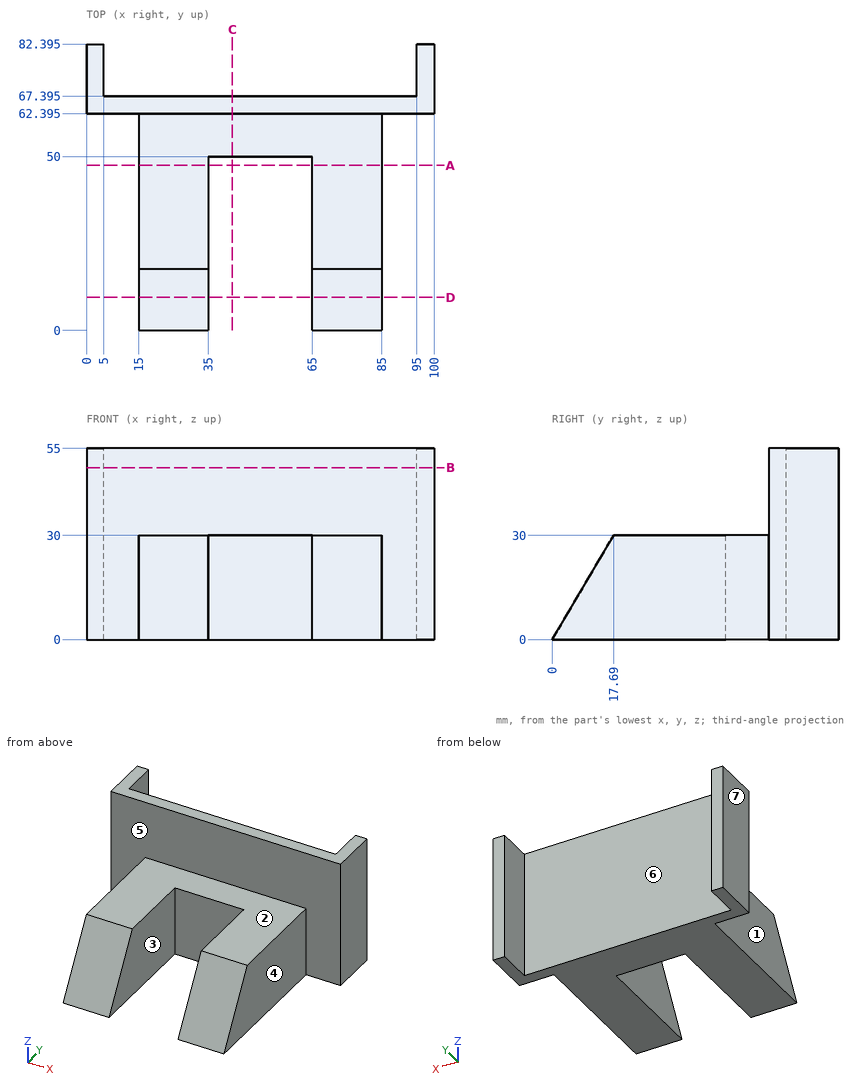
Here's the drawing with two shaded views (mm, measured from the low corner). I have some questions. A direction names the side the tool comes from. Round coordinates to 2 decimals unless told otherwise and drop trailing zeros. Loops run counter-clockwise (first coordinate to the right, second up) from the corner with the lowest first, then second, coordinate; pieces in that order, holes last. Notation, with made-up numbers: (79, 76) -> (129, 76) arc R19 ccw to (129, 86) -> close; hole circle Ø2 at (0, 48). An arc over 180 degrees is marked (long way). Answer as CSV lines item,"result". Start each with the question number.
1. Imagine slicing it at B-B on z = 49.5. Write out the boundary of the cut face in (x, y) (3 decimals).
2. I need wall thicknesses on probe 1 along X at (y, z) = (72, 46.5); probe 2 along X at (y, z) = (17, 23); probe 3 along Y at (x, z) = (61.5, 15) (3 decimals). Which ranges of each line are inside material? Lowest first, please. Write a range as from..to.
3. Imagine slicing it at C-C on x = 42. Write out the boundary of the cut face in (y, z) (3 decimals).
4. Imagine slicing it at A-A on y = 47.5. Write out the boundary of the cut face in (x, z).
5. If we mould it in two halves opening along X, with no side actions, what happens to the marked faces 5, 6 and 7? For each: pulls with the +X half, pulls with the -X half, needs draft (parallel to the pull), parting line crosses it, or undercut.
6. Imagine slicing it at D-D on y = 9.5. Write out the boundary of the cut face in (x, z), plus the area to 3 significant figures.
7. I'm going to push flat-ended pins straight in: P1, Ø16.5, axis at x = 54, z = 35.5, coming from the +Y side (3 decimals); P2, Ø8, axis at x = 71, z = 19, coming from the -Y side (3 decimals); P3, Ø24, axis at y = 15, z = 12.5, coming from the -X side. Where does each tip first touch, or does it pass through?
8. For the marked faces 1, 2, 3 and 4, which set-ups out of +Z, -Z, +X, -X, +Y, -Y let a thin tool reach every point of the face, with its end or its side?
Solution:
1,outline,"(0, 62.395) -> (100, 62.395) -> (100, 82.395) -> (95, 82.395) -> (95, 67.395) -> (5, 67.395) -> (5, 82.395) -> (0, 82.395) -> close"
2,probe 1,"0..5, 95..100"
2,probe 2,"15..35, 65..85"
2,probe 3,"50..67.395"
3,outline,"(50, 0) -> (67.395, 0) -> (67.395, 55) -> (62.395, 55) -> (62.395, 30) -> (50, 30) -> close"
4,outline,"(15, 0) -> (35, 0) -> (35, 30) -> (15, 30) -> close; (65, 0) -> (85, 0) -> (85, 30) -> (65, 30) -> close"
5,face 5,"needs draft"
5,face 6,"undercut"
5,face 7,"pulls with the -X half"
6,outline,"(15, 0) -> (35, 0) -> (35, 16.11) -> (15, 16.11) -> close; (65, 0) -> (85, 0) -> (85, 16.11) -> (65, 16.11) -> close"
6,area,"644 mm²"
7,P1,"y = 67.395"
7,P2,"y = 8.845"
7,P3,"x = 15"
8,face 1,"+Z, -Z, -X, -Y"
8,face 2,"+Z, +X, -X, -Y"
8,face 3,"+Z, -Z, -Y"
8,face 4,"+Z, -Z, +X, -Y"
